```python
from build123d import *

# Parameters (mm, degrees)
F0_W         = 175
F0_H         = 60
F1_DEPTH     = 95
F3_T         = -2.5
F2_W         = 61
F2_H         = 81
F4_DEPTH     = 60.001
F6_D         = 10
F7_W         = 3.5
F7_H         = 3.5
F8_DEPTH     = 60.001
F9_T1_DEPTH  = 116.5
F9_T3_DEPTH  = 78.5
F9_T5_DEPTH  = 78.5
F10_R        = 2.5
F11_T4_DEPTH = 96.25
F12_R        = 2.5
F13_T4_DEPTH = 96.25


# Not quite as in the source:
# - a fillet or chamfer that OpenCascade refuses, or shapes differently, is made with other operations: its cross-section is extruded or revolved along the edge and cut away or added


with BuildPart() as f1:
    # F0 (on Top) → F1 (new body)
    with BuildSketch(Plane.XY):
        Rectangle(F0_W, F0_H)
    extrude(amount=F1_DEPTH)

    # F3
    f3_openings = [f1.faces().sort_by_distance(p)[0] for p in [
        (0, 30, 47.5),
        (0, 0, 0),
    ]]
    offset(amount=F3_T, openings=f3_openings)

    # F2 (on face) → F4 (cut, through all)
    with BuildSketch(Plane.XZ.offset(30)):
        with Locations((0, 54.5)):
            Rectangle(F2_W, F2_H)
    extrude(amount=-F4_DEPTH, mode=Mode.SUBTRACT)

    # F6 (through all)
    with Locations(Plane.XZ.offset(30)):
        with Locations((52.75, 55.5), (52.75, 18), (-52.75, 18), (-52.75, 55.5)):
            Hole(F6_D / 2)

    # F7 (on face) → F8 (cut, through all)
    with BuildSketch(Plane.XZ.offset(30)):
        with Locations((-85.75, 93.25)):
            Rectangle(F7_W, F7_H)
        with Locations((85.75, 93.25)):
            Rectangle(F7_W, F7_H)
    extrude(amount=-F8_DEPTH, mode=Mode.SUBTRACT)

    # F9: fillet of radius 5 on 4 edges, made by hand

    # F9_s2 → F9_t1 (cut)
    with BuildSketch(Plane.XY.offset(-12.5)):
        with BuildLine():
            ThreePointArc((-87.5, -25), (-86.0355339059, -28.5355339059), (-82.5, -30))
            Line((-82.5, -30), (-87.5, -30))
            Line((-87.5, -30), (-87.5, -25))
        make_face()
        with BuildLine():
            ThreePointArc((82.5, -30), (86.0355339059, -28.5355339059), (87.5, -25))
            Line((87.5, -25), (87.5, -30))
            Line((87.5, -30), (82.5, -30))
        make_face()
    extrude(amount=F9_T1_DEPTH, mode=Mode.SUBTRACT)

    # F9_s4 → F9_t3 (cut)
    with BuildSketch(Plane.YZ.offset(-96.5)):
        with BuildLine():
            ThreePointArc((-30, 90), (-28.5355339059, 93.5355339059), (-25, 95))
            Line((-25, 95), (-30, 95))
            Line((-30, 95), (-30, 90))
        make_face()
    extrude(amount=F9_T3_DEPTH, mode=Mode.SUBTRACT)

    # F9_s6 → F9_t5 (cut)
    with BuildSketch(Plane.YZ.offset(18)):
        with BuildLine():
            ThreePointArc((-30, 90), (-28.5355339059, 93.5355339059), (-25, 95))
            Line((-25, 95), (-30, 95))
            Line((-30, 95), (-30, 90))
        make_face()
    extrude(amount=F9_T5_DEPTH, mode=Mode.SUBTRACT)

    # F10
    f10_edges = [f1.edges().sort_by_distance(p)[0] for p in [
        (57.25, -27.5, 92.5),
    ]]
    fillet(f10_edges, radius=F10_R)

    # F11: fillet of radius 2.5 on 1 edges, made by hand


with BuildPart() as f11_tool2:
    # F11_s3 → F11_t4 (new body)
    with BuildSketch(Plane.XY.offset(96.25)):
        with BuildLine():
            ThreePointArc((82.5, -27.5), (84.267766953, -26.767766953), (85, -25))
            Line((85, -25), (85, -27.5))
            Line((85, -27.5), (82.5, -27.5))
        make_face()
    extrude(amount=-F11_T4_DEPTH)

    split(bisect_by=Plane.XY.offset(91.5), keep=Keep.BOTTOM)


with BuildPart() as f1_1:
    add(f1.part)

    # F11_t1: union F11_tool2
    add(f11_tool2.part)

    # F12
    f12_edges = [f1_1.edges().sort_by_distance(p)[0] for p in [
        (-57.25, -27.5, 92.5),
    ]]
    fillet(f12_edges, radius=F12_R)

    # F13: fillet of radius 2.5 on 1 edges, made by hand


with BuildPart() as f13_tool2:
    # F13_s3 → F13_t4 (new body)
    with BuildSketch(Plane.XY):
        with BuildLine():
            ThreePointArc((-82.5, -27.5), (-84.267766953, -26.767766953), (-85, -25))
            Line((-85, -25), (-85, -27.5))
            Line((-85, -27.5), (-82.5, -27.5))
        make_face()
    extrude(amount=F13_T4_DEPTH)

    split(bisect_by=Plane.XY.offset(91.5), keep=Keep.BOTTOM)


with BuildPart() as f1_2:
    add(f1_1.part)

    # F13_t1: union F13_tool2
    add(f13_tool2.part)


solid = f1_2.part
```
Design review of the part built by this model. Coordinates are the model's own, in mm. A direction names the side the tool comes from. Give positions to 0.01 mm unless a question says otherwise; leave off trailing zeros. Order: outer loops, then holes, each group sorted by start corner. A loop starts at its lowest first (then second) coordinate and runs counter-clockwise, first axis right, second up. Notation, with made-up numbers: (86, 75) - (94, 75) arc R22 cw to (94, 99) - close; hole circle Ø7 at (6.5, 39.25). An arc over 180 degrees is marked (long way). Use a Markdown table: item, result. Add a question column.
(1) Machinability: for faces 4 (the face through (57, 3, 92.5)), 5 (the face through (-85, 2, 45)), 6 (the face through (87.5, 2, 45)), 7 (the face through (-30.5, -29, 72)), 8 (the face through (36, -27.5, 44)), which of the approach directions +Z, -Z, +X, -X, +Y, -Y give a long, thin tool a straight path to every point of the face, cutting with its end or side? Answer none if there is none.
(2) Add section C-C on z = 18. Give the boundary of the cut face in (x, y), then the cut area to 3 significant figures.
(3) Add section D-D on z = 73.5. Give the boundary of the cut face in (x, y), then the cut area to 3 significant figures.
(4) Wall thickness on probe 1 along X at (y, z) = (-5.5, 16); probe 2 along Z at (x, y) = (-52.75, -28.7); probe 3 along Z at (x, y) = (52.75, -28.2): over which ranges is each line inside the solid? List them lowest first. Write a range as [from, to].
(5) Mouldability with a two-part tool opening along Z and no side actions: class faces 1 (the face through (57, -29, 93)), 2 (the face through (56.72, -28.73, 14.96)), 3 (the face through (-86.07, -28.5, 45.11)) as +Z half, -Z half, draft (parallel to the pull), parting line (faces both ways), or undercut.
(6) Add section B-B on x = -52.75. Give the boundary of the cut face in (y, z), then the cut area to 3 significant figures.
(7) Clearance check with flat-ended pins moving along their axes: P1, Ø13, axis at x = 52.75, z = 55.5, coming from the +Y side; P2, Ø6, axis at x = 69.5, y = -12, coming from the -Z side; P3, Ø1.1, axis at x = 85.5, y = 11.5, coming from the +Z side. State where each tip first meets the part, or that it passes through.
(8) Add section A-A on y = -8. Give the boundary of the cut face in (x, z), then the cut area to 3 significant figures.
Report:
| question | item | result |
|---|---|---|
| 1 | face 4 | -Z, +X, -X, +Y |
| 1 | face 5 | +Z, -Z, +Y |
| 1 | face 6 | +Z, -Z, +X, +Y, -Y |
| 1 | face 7 | +Z, +Y, -Y |
| 1 | face 8 | -Z, +Y |
| 2 | outline | (-87.5, -25) arc R5 ccw to (-82.5, -30) - (-57.75, -30) - (-57.75, -27.5) - (-82.5, -27.5) arc R2.5 cw to (-85, -25) - (-85, 30) - (-87.5, 30) - close; (-47.75, -30) - (-30.5, -30) - (-30.5, -27.5) - (-47.75, -27.5) - close; (30.5, -30) - (47.75, -30) - (47.75, -27.5) - (30.5, -27.5) - close; (57.75, -30) - (82.5, -30) arc R5 ccw to (87.5, -25) - (87.5, 30) - (85, 30) - (85, -25) arc R2.5 cw to (82.5, -27.5) - (57.75, -27.5) - close |
| 2 | area | 514 mm² |
| 3 | outline | (-87.5, -25) arc R5 ccw to (-82.5, -30) - (-30.5, -30) - (-30.5, -27.5) - (-82.5, -27.5) arc R2.5 cw to (-85, -25) - (-85, 30) - (-87.5, 30) - close; (30.5, -30) - (82.5, -30) arc R5 ccw to (87.5, -25) - (87.5, 30) - (85, 30) - (85, -25) arc R2.5 cw to (82.5, -27.5) - (30.5, -27.5) - close |
| 3 | area | 564 mm² |
| 4 | probe 1 | x = [-87.5, -85], [85, 87.5] |
| 4 | probe 2 | z = [0, 13], [23, 50.5], [60.5, 93.36] |
| 4 | probe 3 | z = [0, 13], [23, 50.5], [60.5, 93.84] |
| 5 | face 1 | +Z half |
| 5 | face 2 | undercut |
| 5 | face 3 | draft |
| 6 | outline | (-30, 0) - (-27.5, 0) - (-27.5, 13) - (-30, 13) - close; (-30, 23) - (-27.5, 23) - (-27.5, 50.5) - (-30, 50.5) - close; (-30, 60.5) - (-27.5, 60.5) - (-27.5, 90) arc R2.5 cw to (-25, 92.5) - (30, 92.5) - (30, 95) - (-25, 95) arc R5 ccw to (-30, 90) - close |
| 6 | area | 327 mm² |
| 7 | P1 | stops at y = -27.5 |
| 7 | P2 | stops at z = 92.5 |
| 7 | P3 | stops at z = 91.5 |
| 8 | outline | (-87.5, 0) - (-85, 0) - (-85, 91.5) - (-87.5, 91.5) - close; (-84, 92.5) - (-30.5, 92.5) - (-30.5, 95) - (-84, 95) - close; (30.5, 92.5) - (84, 92.5) - (84, 95) - (30.5, 95) - close; (85, 0) - (87.5, 0) - (87.5, 91.5) - (85, 91.5) - close |
| 8 | area | 725 mm² |
